Design review of the part built by this model. Coordinates are the model's own, in mm. A direction names the side the tool comes from. Round coordinates to 2 decimals unless told otherwise and drop trailing zeros. Loops run counter-clockwise (first coordinate to the right, second up) from the corner with the lowest first, then second, coordinate; pieces in that order, holes last. Notation, with made-up numbers: (47.25, -25) - (66.25, -25) arc R25 ccw to (66.25, -3) - close; hole circle Ø11 at (82, 35.25). An arc over 180 degrees is marked (long way). Answer as CSV lines item,"result". Start each with the question number.
(1) Mouldability with a two-part tool opening along Y and no side actions: class faces 3 (the flat face through (757, 381, 0)), 4 (the cylindrical face through (887.947, 503.58, -0.089)), 5 (the flat face through (799.162, 457, 0)) as released by +Y, released by -Y, zero draft, split by the parting line, or undercut.
(2) Consider section C-C (z = -0.75). Give the boundary of the cut face in (x, y) (3 decimals).
(3) For faces 1 (the flat face through (1015.062, 457, 0)), 2 (the flat face through (1054, 381, 0)), list the 3-axis set-ups (+Z, -Z, +X, -X, +Y, -Y) from which the entire face can be reached by the end or side of a thin tool; tool diameter is ignored.
(4) For P1, Ø4, axis at x = 1006, z = -3, coming from the -Y side, flat-tipped, find the tip position at first contact; note if it passes through.
(5) Wall thickness on L1, parallel to X at y = 419.5, z = 1.25; L2, parallel to Y at x = 900, z = 1.25; L3, parallel to Y at x = 1005, z = 2: over which ranges is each line inside the solid? List them lowest first.
(6) Consider section A-A (x = 900). Give the boundary of the cut face in (y, z), and give its area (3 significant figures).
(7) Consider section B-B (y = 433). Give the boundary of the cut face in (x, z), and give its area (3 significant figures).
from build123d import *

# Parameters (mm, degrees)
BOSS_EXTRUDE1_DEPTH = 6.35
CAVITY1_START       = -6.35
CAVITY1_OUTLINE_R   = 12.7
CAVITY1_DEPTH       = 12.7
MOVE_FACE_SLOT_BY   = 0.762
MOVE_FACE_SLOT_2_BY = 0.762
MOVE_FACE_SLOT_3_BY = 0.762
MOVE_FACE_SLOT_4_BY = 0.762
MOVE_FACE_SLOT_5_BY = 0.762
MOVE_FACE_SLOT_6_BY = 0.762
MOVE_FACE_HOLE_BY   = 0.635
SLOT_FILLET_R       = 3.175


# Read off the part's stored shape, not the designer's step: Cavity1
with BuildPart() as part:
    # Sketch1 → Boss-Extrude1 (new, symmetric)
    with BuildSketch(Plane.XY):
        Polygon((785.7, 533.4), (785.7, 381), (732.36, 381), (732.36, 685.8), (785.7, 685.8), (1001.6, 685.8), (1087.96, 685.8), (1087.96, 381), (1014.3, 381), (1014.3, 533.4), (1001.6, 533.4), (1001.6, 381), (798.4, 381), (798.4, 533.4), align=None)
    extrude(amount=BOSS_EXTRUDE1_DEPTH, both=True)

    # Cavity1 outline → Cavity1 (cut)
    with BuildSketch(Plane.XY.offset(CAVITY1_START)):
        with Locations((900, 503.049546279)):
            Circle(CAVITY1_OUTLINE_R)
    extrude(amount=CAVITY1_DEPTH, mode=Mode.SUBTRACT)

    # Move Face Slot: a face moved inward by 0.762
    extrude(part.faces().sort_by_distance((1007.95, 533.4, 0))[0], amount=MOVE_FACE_SLOT_BY, dir=(0, 1, 0), mode=Mode.SUBTRACT)

    # Move Face Slot 2: a face moved inward by 0.762
    extrude(part.faces().sort_by_distance((1014.3, 457.2, 0))[0], amount=MOVE_FACE_SLOT_2_BY, dir=(1, 0, 0), mode=Mode.SUBTRACT)

    # Move Face Slot 3: a face moved inward by 0.762
    extrude(part.faces().sort_by_distance((792.05, 533.4, 0))[0], amount=MOVE_FACE_SLOT_3_BY, dir=(0, 1, 0), mode=Mode.SUBTRACT)

    # Move Face Slot 4: a face moved inward by 0.762
    extrude(part.faces().sort_by_distance((798.4, 457.2, 0))[0], amount=MOVE_FACE_SLOT_4_BY, dir=(1, 0, 0), mode=Mode.SUBTRACT)

    # Move Face Slot 5: a face moved inward by 0.762
    extrude(part.faces().sort_by_distance((785.7, 457.2, 0))[0], amount=MOVE_FACE_SLOT_5_BY, dir=(-1, 0, 0), mode=Mode.SUBTRACT)

    # Move Face Slot 6: a face moved inward by 0.762
    extrude(part.faces().sort_by_distance((1001.6, 457.2, 0))[0], amount=MOVE_FACE_SLOT_6_BY, dir=(-1, 0, 0), mode=Mode.SUBTRACT)

    # Move Face Hole: a curved face moved outward by 0.635
    add(Solid.thicken(part.faces().sort_by_distance((887.3, 503.049546279, 0))[0], MOVE_FACE_HOLE_BY))

    # Slot Fillet
    slot_fillet_edges = [part.edges().sort_by_distance(p)[0] for p in [
        (784.938, 381, 0),
        (784.938, 534.162, 0),
        (799.162, 534.162, 0),
        (799.162, 381, 0),
        (1000.838, 381, 0),
        (1000.838, 534.162, 0),
        (1015.062, 534.162, 0),
        (1015.062, 381, 0),
    ]]
    fillet(slot_fillet_edges, radius=SLOT_FILLET_R)


solid = part.part
Determined:
1,face 3,"released by -Y"
1,face 4,"undercut"
1,face 5,"zero draft"
2,outline,"(732.36, 381) - (781.763, 381) arc R3.175 ccw to (784.938, 384.175) - (784.938, 530.987) arc R3.175 cw to (788.113, 534.162) - (795.987, 534.162) arc R3.175 cw to (799.162, 530.987) - (799.162, 384.175) arc R3.175 ccw to (802.337, 381) - (997.663, 381) arc R3.175 ccw to (1000.838, 384.175) - (1000.838, 530.987) arc R3.175 cw to (1004.013, 534.162) - (1011.887, 534.162) arc R3.175 cw to (1015.062, 530.987) - (1015.062, 384.175) arc R3.175 ccw to (1018.237, 381) - (1087.96, 381) - (1087.96, 685.8) - (732.36, 685.8) - close; hole circle Ø24.13 at (900, 503.05)"
3,face 1,"+Z, -Z, -Y"
3,face 2,"+Z, -Z, +X, -X, -Y"
4,P1,"stops at y = 534.16"
5,L1,"x = 732.36 to 784.94, 799.16 to 1000.84, 1015.06 to 1087.96"
5,L2,"y = 381 to 490.98, 515.11 to 685.8"
5,L3,"y = 534.16 to 685.8"
6,outline,"(381, -6.35) - (490.98, -6.35) - (490.98, 6.35) - (381, 6.35) - close; (515.11, -6.35) - (685.8, -6.35) - (685.8, 6.35) - (515.11, 6.35) - close"
6,area,"3,560 mm^2"
7,outline,"(732.36, -6.35) - (784.94, -6.35) - (784.94, 6.35) - (732.36, 6.35) - close; (799.16, -6.35) - (1000.84, -6.35) - (1000.84, 6.35) - (799.16, 6.35) - close; (1015.06, -6.35) - (1087.96, -6.35) - (1087.96, 6.35) - (1015.06, 6.35) - close"
7,area,"4,150 mm^2"
